from build123d import *

# Parameters (mm, degrees)
SKETCH1_R           = 14.7
BOSS_EXTRUDE1_DEPTH = 30
SKETCH2_R           = 19.7
BOSS_EXTRUDE2_DEPTH = 4
SKETCH3_R           = 14.8
BOSS_EXTRUDE3_DEPTH = 20
BOSS_EXTRUDE4_START = -15
BOSS_EXTRUDE4_DEPTH = 15
CHAMFER1_SIZE       = 0.5
CHAMFER2_SIZE       = 1


with BuildPart() as part:
    # Sketch1 → Boss-Extrude1 (new body)
    with BuildSketch(Plane.XY):
        with Locations((-50, 10.3)):
            Circle(SKETCH1_R)
    extrude(amount=-BOSS_EXTRUDE1_DEPTH)

    # Sketch2 → Boss-Extrude2 (add)
    with BuildSketch(Plane.XY):
        with Locations((-50, 10.3)):
            Circle(SKETCH2_R)
    extrude(amount=BOSS_EXTRUDE2_DEPTH)

    # Sketch3 → Boss-Extrude3 (add)
    with BuildSketch(Plane.XY.offset(4)):
        with Locations((-50, 10.3)):
            Circle(SKETCH3_R)
    extrude(amount=BOSS_EXTRUDE3_DEPTH)

    # Sketch5 → Boss-Extrude4 (add)
    with BuildSketch(Plane.XY.offset(24).offset(BOSS_EXTRUDE4_START)):
        with BuildLine():
            Line((-52.3, 24.920191517), (-52.3, 28.420191517))
            Line((-52.3, 28.420191517), (-47.7, 28.420191517))
            Line((-47.7, 28.420191517), (-47.7, 24.920191517))
            ThreePointArc((-47.7, 24.920191517), (-50, 25.1), (-52.3, 24.920191517))
        make_face()
    extrude(amount=BOSS_EXTRUDE4_DEPTH)

    # Chamfer1
    chamfer1_edges = [part.edges().sort_by_distance(p)[0] for p in [
        (-50, 28.420191517, 9),
        (-52.3, 28.420191517, 16.5),
        (-47.7, 28.420191517, 16.5),
        (-50, 28.420191517, 24),
    ]]
    chamfer(chamfer1_edges, length=CHAMFER1_SIZE)

    # Chamfer2
    chamfer2_edges = [part.edges().sort_by_distance(p)[0] for p in [
        (-47.7, 26.420191517, 24),
        (-52.3, 26.420191517, 24),
        (-59.617692031, -0.948999956, 24),
        (-64.7, 10.3, -30),
    ]]
    chamfer(chamfer2_edges, length=CHAMFER2_SIZE - 0.0001)  # a hair under: the kernel refuses the full size


solid = part.part
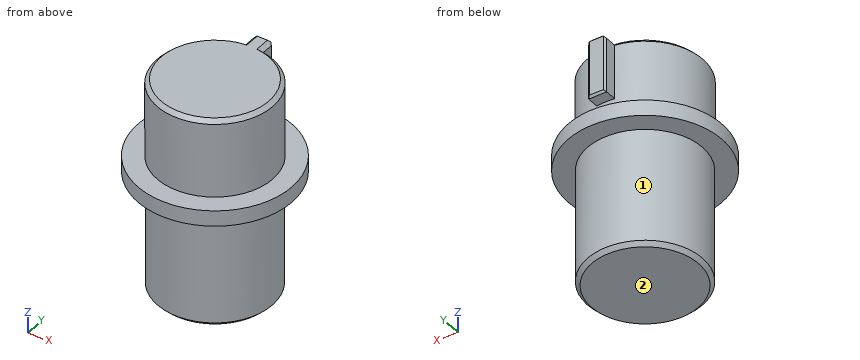
Read the model definition and answer for the solid it produces. Units are mm, in the model's axes. Face numbers are marked on the shaded views. A direction names the side the tool comes from. Give positions to 0.01 mm unless a question says otherwise; leave off trailing zeros. Write each loop counter-clockwise with the first axis right and the second up, starting at its lowest first coordinate (ties: lowest second). Pieces come first, ordered by that corner, then holes. Notation, with made-up numbers: (-8, 85.25) - (8, 85.25) arc R21 cw to (8, 98.25) - close; hole circle Ø5 at (12, -38.75). An arc over 180 degrees is marked (long way). Use CSV: the item, a comma, the result in double quotes. Start each with the question number.
Item 1: The part is cut by section C-C, the plane x = -50. Give the vertices of the cut face in (y, z), and give its area (3 significant figures).
Item 2: For the marked faces 1 and 2, determine the directions among +Z, -Z, +X, -X, +Y, -Y from which every point of the face is accessible in a straight line to the end or side of a thin tool.
Item 3: Consider line 1 (X direction, y = 10.5, z = 17.5); line 2 (Z direction, x = -53.5, y = -7); line 3 (Y direction, x = -38.5, z = 3) (3 decimals). Determine where each line is inside the solid, lowest interval first.
Item 4: Flat-ended cylindrical pins translate along their axes: P1, Ø12, axis at y = 23, z = -10.5, coming from the -X side; P2, Ø3, axis at y = 0.5, z = -2, coming from the +X side; P3, Ø5, axis at x = -35.5, z = 10, coming from the +Y side. Find the tip coordinate at first contact, or state that the pin passes through.
Item 5: The part is cut by section D-D, the plane z = -11.5. Give the vertices of the cut face in (x, y).
Item 6: The part is cut by section B-B, the plane z = 14. Give the vertices of the cut face in (x, y).
Item 7: The part is cut by section A-A, the plane y = 10.3. Give the vertices of the cut face in (x, z).
Taken from the geometry:
1,outline,"(-9.4, 0) - (-4.4, 0) - (-4.4, -29) - (-3.4, -30) - (24, -30) - (25, -29) - (25, 0) - (30, 0) - (30, 4) - (25.1, 4) - (25.1, 9) - (27.92, 9) - (28.42, 9.5) - (28.42, 23.5) - (27.92, 24) - (-3.5, 24) - (-4.5, 23) - (-4.5, 4) - (-9.4, 4) - close"
1,area,"1,680 mm2"
2,face 1,"-Z"
2,face 2,"-Z, +X, -X, +Y, -Y"
3,line 1,"-64.8 to -35.2"
3,line 2,"0 to 4"
3,line 3,"-5.695 to 26.295"
4,P1,"x = -63.08"
4,P2,"x = -37.87"
4,P3,"y = 18.96"
5,outline,"circle Ø29.4 at (-50, 10.3)"
6,outline,"(-52.3, 24.92) arc R14.8 ccw (long way) to (-47.7, 24.92) - (-47.7, 27.92) - (-48.2, 28.42) - (-51.8, 28.42) - (-52.3, 27.92) - close"
7,outline,"(-69.7, 0) - (-64.7, 0) - (-64.7, -29) - (-63.7, -30) - (-36.3, -30) - (-35.3, -29) - (-35.3, 0) - (-30.3, 0) - (-30.3, 4) - (-35.2, 4) - (-35.2, 23) - (-36.2, 24) - (-63.8, 24) - (-64.8, 23) - (-64.8, 4) - (-69.7, 4) - close"
